Work out the finished part from the listing and answer in its coordinate system (mm). Coordinates: 2 decimals unless noted, no trailing zeros. Order: outer loops, then holes, each group sorted by start corner. A loop starts at its lowest first (then second) coordinate and runs counter-clockwise, first axis right, second up.
1. The part is cut by section B-B, the plane x = 17. Give the vertices of the cut face in (y, z) (3 decimals), then the cut area to 3 significant figures.
2. The part is cut by section D-D, the plane z = -19. Give the vertices of the cut face in (x, y), then the cut area to 3 significant figures.
3. The part is cut by section A-A, the plane z = 0. Give the vertices of the cut face in (x, y), then the cut area to 4 significant figures.
4. Find the intervals of material crossed by probe 1 along X at (y, z) = (0.65, -18.5); probe 2 along Z at (x, y) = (-8, 1.45); probe 3 along Z at (x, y) = (18, 0.8), in increasing order.
5. Flat-ended cylindrical pins translate along their axes: pin 1 Ø1.5 at (x, z) = (7.5, -18.5) entering from +Y; pin 2 Ø0.7 at (x, y) = (7.5, 1) entering from +Z; pin 3 Ø1 at (y, z) = (1, -17.5) entering from -X (3 decimals); pin 4 Ø0.9 at (y, z) = (0.5, -19.5) entering from -X. Find the tip coordinate at first contact, or state that the pin passes through.
6. The part is cut by section C-C, the plane y = 1.45. Give the vertices of the cut face in (x, z).
```python
from build123d import *

# Parameters (mm, degrees)
BOSS_EXTRUDE1_DEPTH = 1.75
FILLET2_R           = 2
FILLET3_R           = 3
SKETCH2_R           = 1.2500000000000004
SKETCH2_R_2         = 1.2499999999999996
CUT_EXTRUDE1_DEPTH  = 1.75


with BuildPart() as part:
    # Sketch1 → Boss-Extrude1 (new body)
    with BuildSketch(Plane(origin=(0, 0, 0), x_dir=(1, 0, 0), z_dir=(0, 1, 0))):
        with BuildLine():
            Line((-4, 23.410734717218936), (-4, 19.03424545391805))
            Line((-4, 19.03424545391805), (-3.999999999999999, 15))
            Line((-3.999999999999999, 15), (-9, 15))
            Line((-9, 15), (-9, 17.242462121170515))
            ThreePointArc((-9, 17.242462121170515), (-3.57e-15, -19.45), (9, 17.242462121170515))
            Line((9, 17.242462121170515), (9.000000000000002, 15))
            Line((9.000000000000002, 15), (4, 15))
            Line((4, 15), (4, 19.034245453918047))
            Line((4, 19.034245453918047), (3.999999999999999, 23.410734717218936))
            ThreePointArc((3.999999999999999, 23.410734717218936), (-4.36e-15, -23.75), (-4, 23.410734717218936))
        make_face()
    extrude(amount=BOSS_EXTRUDE1_DEPTH)

    # Fillet2
    # the kernel refuses this fillet: 2 mm, written as the material it adds along each edge
    with BuildSketch(Plane(origin=(9.000000000000005, 0, -17.24246212117051), x_dir=(-2.38e-15, 0, 1), z_dir=(0, 1, 0))) as fillet2_piece_1:
        with BuildLine():
            CenterArc((3.4030154331547133, 1.62883885330701), FILLET2_R, 142.4753629283073, 92.05463357157004)
            Line((1.8168324316629296, 2.8470438794739996), (1.7851087716330947, 2.871407979997339))
            ThreePointArc((1.7851087716330947, 2.871407979997339), (0.812783961312924, 1.4845493734112696), (-0.0354600763417388, 0.01850899742930592))
            Line((-0.0354600763417388, 0.01850899742930592), (1e-16, -0.03999999999999915))
            ThreePointArc((1e-16, -0.03999999999999915), (1.1212310605852558, -0.04000000000000004), (2.219251054930826, -0.03257677706614009))
            Line((2.219251054930826, -0.03257677706614009), (2.24246212117051, 0))
        make_face()
    extrude(amount=1.75)
    with BuildSketch(Plane(origin=(-9, 0, -17.242462121170515), x_dir=(-0.842979895323632, 0, 0.5379450679020662), z_dir=(0, 1, 0))) as fillet2_piece_2:
        with BuildLine():
            CenterArc((3.203713774320002, 1.9924477660817068), FILLET2_R, 182.92614352023125, 92.05463357157015)
            Line((1.2063214380408842, 1.8903504841715306), (1.1663735913153022, 1.8883085385333274))
            ThreePointArc((1.1663735913153022, 1.8883085385333274), (0.5694415232074965, 0.966693044801846), (-0.03371919581294457, 0.02151780271608219))
            Line((-0.03371919581294457, 0.02151780271608219), (-0.00347286045996735, -0.03984895532163413))
            ThreePointArc((-0.00347286045996735, -0.03984895532163413), (1.68867839865919, -0.11344547485539745), (3.380829657778342, -0.03984895532163431))
            Line((3.380829657778342, -0.03984895532163431), (3.3773567973183756, 1.9e-16))
        make_face()
    extrude(amount=1.75)

    # Fillet3
    fillet3_edges = [part.edges().sort_by_distance(p)[0] for p in [
        (-9, 0.875, -15),
        (9.000000000000002, 0.875, -15),
        (4, 0.875, -15),
        (-3.999999999999999, 0.875, -15),
    ]]
    fillet(fillet3_edges, radius=FILLET3_R)

    # Sketch2 → Cut-Extrude1 (cut)
    with BuildSketch(Plane(origin=(0, 1.75, 0), x_dir=(1, 0, 0), z_dir=(0, 1, 0))):
        with Locations(Location((-7.5, 18.5, 0), (0, 0, 270))):
            Circle(SKETCH2_R)
        with Locations(Location((7.5, 18.5, 0), (0, 0, 270))):
            Circle(SKETCH2_R_2)
    extrude(amount=-CUT_EXTRUDE1_DEPTH, mode=Mode.SUBTRACT)


solid = part.part
```
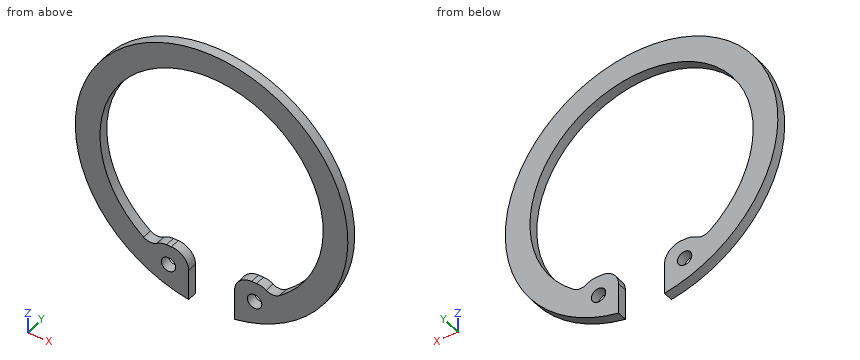
Geometry says:
1. outline: (0, -16.585) - (1.75, -16.585) - (1.75, -9.45) - (0, -9.45) - close; (0, 9.45) - (1.75, 9.45) - (1.75, 16.585) - (0, 16.585) - close
1. area: 25.0 mm2
2. outline: (-14.25, 0) - (-8.65, 0) - (-8.65, 1.75) - (-14.25, 1.75) - close; (-6.35, 0) - (-4, 0) - (-4, 1.75) - (-6.35, 1.75) - close; (4, 0) - (6.35, 0) - (6.35, 1.75) - (4, 1.75) - close; (8.65, 0) - (14.25, 0) - (14.25, 1.75) - (8.65, 1.75) - close
2. area: 27.9 mm2
3. outline: (-23.75, 0) - (-19.45, 0) - (-19.45, 1.75) - (-23.75, 1.75) - close; (19.45, 0) - (23.75, 0) - (23.75, 1.75) - (19.45, 1.75) - close
3. area: 15.05 mm2
4. probe 1: x = -14.89 to -8.75, -6.25 to -4, 4 to 6.25, 8.75 to 14.89
4. probe 2: z = -22.36 to -19.65, -17.35 to -15, 17.73 to 22.36
4. probe 3: z = -15.49 to -7.37, 7.37 to 15.49
5. pin 1: passes through
5. pin 2: stops at z = 22.65
5. pin 3: stops at x = -16.585
5. pin 4: stops at x = -14.18
6. outline: (-11.85, -15.43) arc R19.45 cw (long way) to (11.85, -15.43) arc R2 cw to (9.52, -15.5) arc R3 ccw to (7.86, -15) - (7, -15) arc R3 ccw to (4, -18) - (4, -23.41) arc R23.75 ccw (long way) to (-4, -23.41) - (-4, -18) arc R3 ccw to (-7, -15) - (-7.86, -15) arc R3 ccw to (-9.52, -15.5) arc R2 cw to start; hole circle Ø2.5 at (-7.5, -18.5); hole circle Ø2.5 at (7.5, -18.5)
